For this review, take the finished solid that the model builds, in its own axes (mm). A direction names the side the tool comes from. Round coordinates to 2 decimals unless told otherwise and drop trailing zeros. Order: outer loops, then holes, each group sorted by start corner. A loop starts at its lowest first (then second) coordinate and runs counter-clockwise, first axis right, second up. Notation, with made-up numbers: (86, 41) -> (134, 41) arc R15 ccw to (134, 66) -> close; hole circle Ø4 at (-16.75, -11). An arc over 180 degrees is marked (long way). Use a Markdown table: item, result. Add a question column.
1) Consider section C-C (y = 30). State the section outline as (x, z) points.
2) Consider section A-A (z = 23). State the section outline as (x, y) points, plus the area to 3 significant figures.
3) Draft analysis for pull direction X (two halves, no side actions). For faces 1 (the face through (25.85, 21, 12)), 2 (the face through (15.2, 27.5, 34.3)), 3 (the face through (28.85, 21, 18)), state which applies: pulls with the +X half, pulls with the -X half, needs draft (parallel to the pull), parting line crosses it, or undercut.
4) Wall thickness on line 1 along Y through (x, z) = (7, 20.5); line 2 along X through (y, z) = (30.5, 6); line 3 along Y through (x, z) = (6.25, 32): over which ranges is each line inside the solid? List them lowest first. Write a range as [from, to].
5) Machinability: for faces 4 (the face through (15.161, 18.882, 36.003)), 5 (the face through (4.85, 21, 12)), which of the approach directions +Z, -Z, +X, -X, +Y, -Y give a long, thin tool a straight path to every point of the face, cutting with its end or side? Answer none if there is none.
```python
from build123d import *

# Parameters (mm, degrees)
F0_W     = 27
F0_H     = 37
F0_W_2   = 21
F0_H_2   = 31
F1_DEPTH = 25
F2_W     = 27
F2_H     = 37
F3_DEPTH = 12
F4_SIZE2 = 8
F4_SIZE  = 15
F5_R     = 5
F6_R     = 1
F7_DEPTH = 27.001
F8_R     = 1


with BuildPart() as f1:
    # F0 (on Top) → F1 (new body)
    with BuildSketch(Plane.XY):
        with Locations((15.3503448237, 21.0609438564)):
            Rectangle(F0_W, F0_H)
        with Locations((15.3503448237, 21.0609438564)):
            Rectangle(F0_W_2, F0_H_2, mode=Mode.SUBTRACT)
    extrude(amount=F1_DEPTH)

    # F2 (on face) → F3 (join)
    with BuildSketch(Plane.XY.offset(25)):
        with Locations((15.3503448237, 21.0609438564)):
            Rectangle(F2_W, F2_H)
    extrude(amount=F3_DEPTH)

    # F4
    f4_edges = [f1.edges().sort_by_distance(p)[0] for p in [
        (15.350345, 39.560944, 37),
        (15.350345, 2.560944, 37),
    ]]
    f4_side = f1.faces().sort_by_distance((15.350345, 21.060944, 37))[0]
    chamfer(f4_edges, length=F4_SIZE, length2=F4_SIZE2, reference=f4_side)

    # F5
    f5_edges = [f1.edges().sort_by_distance(p)[0] for p in [
        (15.350345, 24.560944, 37),
        (15.350345, 17.560944, 37),
    ]]
    fillet(f5_edges, radius=F5_R)

    # F6 (on face) → F7 (cut, through all)
    with BuildSketch(Plane(origin=(1.8503448237, 0, 0), x_dir=(0, -1, 0), z_dir=(-1, 0, 0))):
        with Locations((-32.6124144447, 32.7058823529)):
            Circle(F6_R)
        with Locations((-9.5094732682, 32.7058823529)):
            Circle(F6_R)
        with Locations((-25.6638850329, 36.4117647059)):
            Circle(F6_R)
        with Locations((-16.45800268, 36.4117647059)):
            Circle(F6_R)
        with Locations((-30.2415320917, 33.9703529412)):
            Circle(F6_R)
        with Locations((-11.8803556211, 33.9703529412)):
            Circle(F6_R)
        with Locations((-18.8109438564, 37)):
            Circle(F6_R)
        with Locations((-23.3109438564, 37)):
            Circle(F6_R)
        with Locations((-4.7668262094, 30.1764705882)):
            Circle(F6_R)
        with Locations((-37.3550615035, 30.1764705882)):
            Circle(F6_R)
        with Locations((-7.1377085623, 31.4409411765)):
            Circle(F6_R)
        with Locations((-34.9841791505, 31.4409411765)):
            Circle(F6_R)
        with Locations((-27.9527085623, 35.1910588235)):
            Circle(F6_R)
        with Locations((-14.1691791505, 35.1910588235)):
            Circle(F6_R)
    extrude(amount=-F7_DEPTH, mode=Mode.SUBTRACT)

    # F8
    f8_edges = [f1.edges().sort_by_distance(p)[0] for p in [
        (28.850345, 39.560944, 14.5),
        (1.850345, 39.560944, 14.5),
        (28.850345, 2.560944, 14.5),
        (1.850345, 2.560944, 14.5),
    ]]
    fillet(f8_edges, radius=F8_R)


solid = f1.part
```
Results list:
| question | item | result |
|---|---|---|
| 1 | outline | (1.85, 0) -> (4.85, 0) -> (4.85, 25) -> (25.85, 25) -> (25.85, 0) -> (28.85, 0) -> (28.85, 33) -> (1.85, 33) -> close |
| 2 | outline | (1.85, 3.56) arc R1 ccw to (2.85, 2.56) -> (27.85, 2.56) arc R1 ccw to (28.85, 3.56) -> (28.85, 38.56) arc R1 ccw to (27.85, 39.56) -> (2.85, 39.56) arc R1 ccw to (1.85, 38.56) -> close; hole (4.85, 5.56) -> (25.85, 5.56) -> (25.85, 36.56) -> (4.85, 36.56) -> close |
| 2 | area | 347 mm2 |
| 3 | face 1 | undercut |
| 3 | face 2 | needs draft |
| 3 | face 3 | pulls with the +X half |
| 4 | line 1 | [2.56, 5.56], [36.56, 39.56] |
| 4 | line 2 | [1.85, 4.85], [25.85, 28.85] |
| 4 | line 3 | [8.19, 8.8], [10.22, 31.9], [33.32, 33.94] |
| 5 | face 4 | +Z, +X, -X |
| 5 | face 5 | -Z |
